Build history of the part. All positions in model axes, mm. A direction names the side the tool comes from. Round coordinates to 2 decimals unless told otherwise and drop trailing zeros. Loops run counter-clockwise (first coordinate to the right, second up) from the corner with the lowest first, then second, coordinate; pieces in that order, holes last.
Autodesk Inventor part; units mm, degrees
ref_plane "YZ Plane" through (0, 0, 0) normal (1, 0, 0) x (0, 1, 0)
ref_plane "XZ Plane" through (0, 0, 0) normal (0, 1, 0) x (-1, 0, 0)
ref_plane "XY Plane" through (0, 0, 0) normal (0, 0, 1) x (1, 0, 0)
sketch "Sketch_1" plane through (0, 0, 0) normal (1, 0, 0) x (0, 1, 0)
  line L0 (0, 76.2) -> (0, 0)
  line L1 (0, 0) -> (76.2, 0)
  arc A0 (76.2, 0) -> (71.4248, 4.7752) centre (71.4248, 0) ccw
  line L2 (71.4248, 4.7752) -> (7.9502, 4.7752)
  arc A1 (4.7752, 7.9502) -> (7.9502, 4.7752) centre (7.9502, 7.9502) ccw
  line L3 (4.7752, 7.9502) -> (4.7752, 71.4248)
  arc A2 (4.7752, 71.4248) -> (0, 76.2) centre (0, 71.4248) ccw
extrude "Extrusion1" add sketch "Sketch_1" along normal mid plane 47.625
sketch "Sketch2" plane through (23.8125, 0, 0) normal (0, 0, -1) x (-1, 0, 0)
  point P0 (11.1125, 63.5)
hole "Hole1" at (12.7, 63.5, 0) direction (0, 0, 1) diameter 7.1374 depth 5.2527
sketch "Sketch3" plane through (23.8125, 0, 0) normal (0, 0, -1) x (-1, 0, 0)
  point P0 (36.5125, 38.1)
hole "Hole2" at (-12.7, 38.1, 0) direction (0, 0, 1) diameter 7.1374 depth 5.2527
sketch "Sketch4" plane through (23.8125, 0, 0) normal (0, 0, -1) x (-1, 0, 0)
  point P0 (36.5125, 63.5)
hole "Hole3" at (-12.7, 63.5, 0) direction (0, 0, 1) diameter 7.1374 depth 5.2527
sketch "Sketch5" plane through (-23.8125, 0, 76.2) normal (0, -1, 0) x (1, 0, 0)
  point P0 (36.5125, -38.1)
hole "Hole4" at (12.7, 0, 38.1) direction (0, 1, 0) diameter 7.1374 depth 5.2527
sketch "Sketch6" plane through (-23.8125, 0, 76.2) normal (0, -1, 0) x (1, 0, 0)
  point P0 (36.5125, -12.7)
hole "Hole5" at (12.7, 0, 63.5) direction (0, 1, 0) diameter 7.1374 depth 5.2527
sketch "Sketch7" plane through (-23.8125, 0, 76.2) normal (0, -1, 0) x (1, 0, 0)
  point P0 (11.1125, -38.1)
hole "Hole6" at (-12.7, 0, 38.1) direction (0, 1, 0) diameter 7.1374 depth 5.2527
sketch "Sketch8" plane through (-23.8125, 0, 76.2) normal (0, -1, 0) x (1, 0, 0)
  point P0 (11.1125, -12.7)
hole "Hole7" at (-12.7, 0, 63.5) direction (0, 1, 0) diameter 7.1374 depth 5.2527
sketch "Sketch9" plane through (23.8125, 0, 0) normal (0, 0, -1) x (-1, 0, 0)
  point P0 (11.1125, 38.1)
hole "Hole8" at (12.7, 38.1, 0) direction (0, 0, 1) diameter 7.1374 depth 5.2527
sketch "Sketch10" plane through (23.8125, 0, 0) normal (0, 0, -1) x (-1, 0, 0)
  point P0 (11.1125, 12.7)
hole "Hole9" at (12.7, 12.7, 0) direction (0, 0, 1) diameter 7.1374 depth 5.2527
sketch "Sketch11" plane through (23.8125, 0, 0) normal (0, 0, -1) x (-1, 0, 0)
  point P0 (36.5125, 12.7)
hole "Hole10" at (-12.7, 12.7, 0) direction (0, 0, 1) diameter 7.1374 depth 5.2527
sketch "Sketch12" plane through (-23.8125, 0, 76.2) normal (0, -1, 0) x (1, 0, 0)
  point P0 (36.5125, -63.5)
hole "Hole11" at (12.7, 0, 12.7) direction (0, 1, 0) diameter 7.1374 depth 5.2527
sketch "Sketch13" plane through (-23.8125, 0, 76.2) normal (0, -1, 0) x (1, 0, 0)
  point P0 (11.1125, -63.5)
hole "Hole12" at (-12.7, 0, 12.7) direction (0, 1, 0) diameter 7.1374 depth 5.2527
properties part number "4014"
(1) Pin check, flat tips, straight feed: P1, Ø4.5, axis at x = 12.7, y = 63.5, coming from the -Z side; P2, Ø12, axis at x = 17, y = 62.5, coming from the +Z side; P3, Ø11.5, axis at x = -12.7, y = 12.7, coming from the +Z side; P4, Ø14.5, axis at x = 4.5, z = 40, coming from the +Y side. Stop position of each tip, or through.
Responses:
P1: passes through
P2: stops at z = 4.78
P3: stops at z = 4.94
P4: stops at y = 4.78
(2) Which spindle directions (+Z, -Z, +X, -X, +Y, -Y) get a long thin tool onto all of the face, cutting with end or side? Do faces 1 (the face through (0, 4.775, 39)), 2 (the face through (-12.857, 59.935, 2.421)). Say none if no direction does.
Responses:
face 1: +Z, +X, -X, +Y
face 2: +Z, -Z
(3) Probe line 1 (X direction, y = 3, z = 38); line 2 (Y direction, x = -12.7, z = 2.4); line 3 (X direction, y = 12, z = 3). List the from-to ranges inside material, lowest first.
Responses:
line 1: x = -23.81 to -16.27, -9.13 to 9.13, 16.27 to 23.81
line 2: y = 0 to 9.13, 16.27 to 34.53, 41.67 to 59.93, 67.07 to 75.55
line 3: x = -23.81 to -16.2, -9.2 to 9.2, 16.2 to 23.81
(4) Pull direction Z, two halves, no side cores. Call faces 3 (the face through (12.543, 2.421, 67.065)), 4 (the face through (-0.33, 3.34, 74.84)), 5 (the face through (-9.216, 37.326, 2.421)): +Z half, -Z half, draft (parallel to the pull), parting line (faces both ways), or undercut.
Responses:
face 3: undercut
face 4: +Z half
face 5: draft
(5) Slice it at C-C on x = 12.7. Count the separate pieces of the cut face and the enclosed holes in it, plus the area to 3 significant figures.
Responses:
separate pieces: 7
enclosed holes: 0
area: 493 mm2
(6) Slice it at A-A on z = 63.5. List the corners of the cut face in (x, y), plus the area to 3 significant figures.
Responses:
outline: (-23.81, 0) - (-16.27, 0) - (-16.27, 4.78) - (-23.81, 4.78) - close; (-9.13, 0) - (9.13, 0) - (9.13, 4.78) - (-9.13, 4.78) - close; (16.27, 0) - (23.81, 0) - (23.81, 4.78) - (16.27, 4.78) - close
area: 159 mm2
(7) Slice it at D-D on x = 19.5. List the corners of the cut face in (y, z) (3 decimals).
Responses:
outline: (0, 0) - (76.2, 0) arc R4.775 ccw to (71.425, 4.775) - (7.95, 4.775) arc R3.175 cw to (4.775, 7.95) - (4.775, 71.425) arc R4.775 ccw to (0, 76.2) - close
